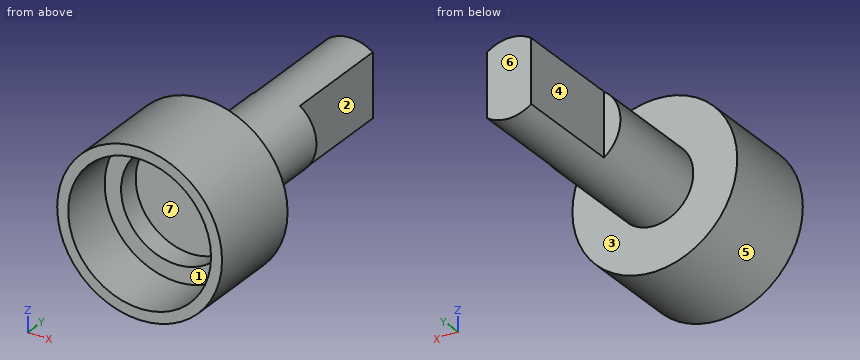
```python
from build123d import *

# Parameters (mm, degrees)
SKETCH1_R           = 1.75
BOSS_EXTRUDE1_DEPTH = 10
CUT_EXTRUDE1_DEPTH  = 5
SKETCH3_R           = 3.75
BOSS_EXTRUDE2_DEPTH = 4.5
SKETCH4_R           = 3.25
CUT_EXTRUDE2_DEPTH  = 2.5
SKETCH5_R           = 2.5
CUT_EXTRUDE3_DEPTH  = 1


with BuildPart() as part:
    # Sketch1 → Boss-Extrude1 (new body)
    with BuildSketch(Plane(origin=(0, 0, 0), x_dir=(1, 0, 0), z_dir=(0, 1, 0))):
        Circle(SKETCH1_R)
    extrude(amount=BOSS_EXTRUDE1_DEPTH)

    # Sketch2 → Cut-Extrude1 (cut)
    with BuildSketch(Plane(origin=(0, 10, 0), x_dir=(1, 0, 0), z_dir=(0, 1, 0))):
        with BuildLine():
            Line((-1, 1.436140662), (-1, -1.436140662))
            ThreePointArc((-1, -1.436140662), (-1.75, 0), (-1, 1.436140662))
        make_face()
        with BuildLine():
            Line((1, 1.436140662), (1, -1.436140662))
            ThreePointArc((1, -1.436140662), (1.75, 0), (1, 1.436140662))
        make_face()
    extrude(amount=-CUT_EXTRUDE1_DEPTH, mode=Mode.SUBTRACT)

    # Sketch3 → Boss-Extrude2 (add)
    with BuildSketch(Plane.XZ):
        Circle(SKETCH3_R)
    extrude(amount=BOSS_EXTRUDE2_DEPTH)

    # Sketch4 → Cut-Extrude2 (cut)
    with BuildSketch(Plane.XZ.offset(4.5)):
        Circle(SKETCH4_R)
    extrude(amount=-CUT_EXTRUDE2_DEPTH, mode=Mode.SUBTRACT)

    # Sketch5 → Cut-Extrude3 (cut)
    with BuildSketch(Plane.XZ.offset(2)):
        Circle(SKETCH5_R)
    extrude(amount=-CUT_EXTRUDE3_DEPTH, mode=Mode.SUBTRACT)


solid = part.part
```
CAD build for the part. Positions are in the model's coordinates, mm. Face numbers are marked on the shaded views. A direction names the side the tool comes from. Give positions to 0.01 mm unless a question says otherwise; leave off trailing zeros. Write each loop counter-clockwise with the first axis right and the second up, starting at its lowest first coordinate (ties: lowest second). Pieces come first, ordered by that corner, then holes. Notation, with made-up numbers: M 45.5,67 L 101.5,67 A17 ccw 101.5,91 Z; hole C 67,44.25 d8. An arc over 180 degrees is marked long. Return JSON: item names as keys, results as strings. Group by question number.
(1) Flat gauge pins, fed straight in: pin 1 Ø4 at (x, z) = (0, 0) entering from -Y; pin 2 Ø3 at (y, z) = (8, 0.5) entering from +X; pin 3 Ø1.5 at (x, y) = (-1.5, 8) entering from -Z. Where does each tip first touch, or does it go through?
(2) Band-saw the part on D-D (y = 6.5). Give the cut face in (x, z).
(3) Mould opens along Z. For the marked faces 5, 6 and 7 say: pulls with the +Z half, pulls with the -Z half, needs draft (parallel to the pull), parting line crosses it, or undercut.
(4) Band-saw the part on C-C (z = 0). Give the cut face in (x, y), and give its area (3 significant figures).
(5) Drill centre lines: L1, parallel to Z at x = 0, y = -1.6; L2, parallel to Z at x = 0, y = -2.6; L3, parallel to Z at x = -1, y = 1. Where is each one in solid material? Low to high. Write a range as [from, to].
(6) Band-saw the part on B-B (y = -1.75). Give the cut face in (x, z).
(7) 3-axis set-ups, long thin cutter, end or side, ignore diameter. For the marked faces 1, 2, 3 and 4: which of +Z, -Z, +X, -X, +Y, -Y reach the whole face in a straight line?
(8) Band-saw the part on A-A (x = 0). Give the cut face in (y, z), and give its area (3 significant figures).
Entries:
{
 "1": {"pin 1": "stops at y = -1", "pin 2": "stops at x = 1", "pin 3": "stops at z = -1.58"},
 "2": {"outline": "M -1,-1.44 A1.75 ccw 1,-1.44 L 1,1.44 A1.75 ccw -1,1.44 Z"},
 "3": {"face 5": "parting line crosses it", "face 6": "needs draft", "face 7": "undercut"},
 "4": {"outline": "M -3.75,-4.5 L -3.25,-4.5 L -3.25,-2 L -2.5,-2 L -2.5,-1 L 2.5,-1 L 2.5,-2 L 3.25,-2 L 3.25,-4.5 L 3.75,-4.5 L 3.75,0 L 1.75,0 L 1.75,5 L 1,5 L 1,10 L -1,10 L -1,5 L -1.75,5 L -1.75,0 L -3.75,0 Z", "area": "40.0 mm^2"},
 "5": {"L1": "z = [-3.75, -2.5], [2.5, 3.75]", "L2": "z = [-3.75, -3.25], [3.25, 3.75]", "L3": "z = [-1.44, 1.44]"},
 "6": {"outline": "C 0,0 d7.5; hole C 0,0 d5"},
 "7": {"face 1": "-Y", "face 2": "+Z, -Z, +X, +Y", "face 3": "+Y", "face 4": "+Z, -Z, -X, +Y"},
 "8": {"outline": "M -4.5,-3.75 L 0,-3.75 L 0,-1.75 L 10,-1.75 L 10,1.75 L 0,1.75 L 0,3.75 L -4.5,3.75 L -4.5,3.25 L -2,3.25 L -2,2.5 L -1,2.5 L -1,-2.5 L -2,-2.5 L -2,-3.25 L -4.5,-3.25 Z", "area": "47.5 mm^2"}
}
